Check sheet for the modelled part. Datum: model origin and axes. Units: mm. Face numbers are marked on the shaded views. A direction names the side the tool comes from. Round coordinates to 2 decimals unless told otherwise and drop trailing zeros. Order: outer loops, then holes, each group sorted by start corner. A loop starts at its lowest first (then second) coordinate and runs counter-clockwise, first axis right, second up.
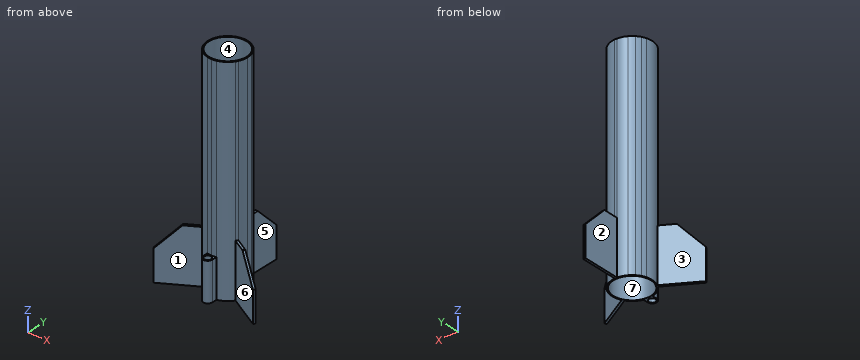
from build123d import *

# Parameters (mm, degrees)
F0_R     = 12.25
F1_DEPTH = 140
F2_DEPTH = 35
F3_SIZE  = 15
F4_COUNT = 3
F0_R_2   = 2.25
F5_DEPTH = 25
F6_START = 62
F0_R_3   = 11
F6_DEPTH = 2


with BuildPart() as f1:
    # F0 (on Top) → F1 (new body)
    with BuildSketch(Plane.XY):
        with BuildLine():
            ThreePointArc((3, -12.6491106407), (10.1980390272, -8.0622577483), (13, 0))
            ThreePointArc((13, 0), (9.4538352006, 8.9232841488), (0.75, 12.9783473524))
            ThreePointArc((0.75, 12.9783473524), (0, 13), (-0.75, 12.9783473524))
            ThreePointArc((-0.75, 12.9783473524), (-12.9501843924, 1.1369803002), (-3, -12.6491106407))
            ThreePointArc((-3, -12.6491106407), (-1.5102254126, -12.9119796779), (2.58e-08, -13))
            ThreePointArc((2.58e-08, -13), (1.5102254382, -12.9119796749), (3, -12.6491106407))
        make_face()
        Circle(F0_R, mode=Mode.SUBTRACT)
    extrude(amount=F1_DEPTH)

    # F0 (on Top) → F2 (join)
    with BuildSketch(Plane.XY):
        with BuildLine():
            ThreePointArc((-0.75, 12.9783473524), (0, 13), (0.75, 12.9783473524))
            Line((0.75, 12.9783473524), (0.75, 37.9783473524))
            Line((0.75, 37.9783473524), (-0.75, 37.9783473524))
            Line((-0.75, 37.9783473524), (-0.75, 12.9783473524))
        make_face()
    extrude(amount=F2_DEPTH)

    # F3
    f3_edges = [f1.edges().sort_by_distance(p)[0] for p in [
        (0, 37.978347, 35),
    ]]
    chamfer(f3_edges, length=F3_SIZE)


with BuildPart() as f4_1:
    # F4: instance of F1
    add(f1.part.rotate(Axis((0, 0, 140), (0, 0, 1)), 1 * 360 / F4_COUNT))


with BuildPart() as f4_2:
    # F4: instance of F1
    add(f1.part.rotate(Axis((0, 0, 140), (0, 0, 1)), 2 * 360 / F4_COUNT))


with BuildPart() as f1_1:
    add(f1.part)

    add(f4_1.part)  # F5 merges F4_1

    add(f4_2.part)  # F5 merges F4_2
    # F0 (on Top) → F5 (join)
    with BuildSketch(Plane.XY):
        with BuildLine():
            ThreePointArc((3, -16), (2.1213203527, -13.8786796655), (2.58e-08, -13))
            ThreePointArc((2.58e-08, -13), (-2.1213203345, -13.8786796473), (-3, -16))
            ThreePointArc((-3, -16), (0, -19), (3, -16))
        make_face()
        with Locations((0, -16)):
            Circle(F0_R_2, mode=Mode.SUBTRACT)
        with BuildLine():
            Line((3, -16), (3, -12.6491106407))
            ThreePointArc((3, -12.6491106407), (1.5102254382, -12.9119796749), (2.58e-08, -13))
            ThreePointArc((2.58e-08, -13), (2.1213203527, -13.8786796655), (3, -16))
        make_face()
        with BuildLine():
            ThreePointArc((-3, -16), (-2.1213203345, -13.8786796473), (2.58e-08, -13))
            ThreePointArc((2.58e-08, -13), (-1.5102254126, -12.9119796779), (-3, -12.6491106407))
            Line((-3, -12.6491106407), (-3, -16))
        make_face()
    extrude(amount=F5_DEPTH)

    # F0 (on Top) → F6 (join)
    with BuildSketch(Plane.XY.offset(F6_START)):
        Circle(F0_R)
        Circle(F0_R_3, mode=Mode.SUBTRACT)
    extrude(amount=F6_DEPTH)


solid = f1_1.part
1) Gauge pin test, flat ends, axial feed: pin 1 (20 mm diameter, centred on y = 26.5, z = 23.5, fed in from +X); pin 2 (5 mm diameter, centred on x = -14.5, y = -10, fed in from +Z); pin 3 (1.8 mm diameter, centred on x = -0.5, y = -16, fed in from +Z); pin 4 (1 mm diameter, centred on y = -14, z = 16.5, fed in from +X). Record the tip position at first contact, or that the pin passes through.
2) Scan lines: line 1 (Y direction, x = 1, z = 22.5); line 2 (X direction, y = 1, z = 9); line 3 (Y direction, x = -2, z = 11). Record each from-to range of solid material in increasing order.
3) Set-up check for the marked faces 1, 2, 3 and 4: record each of +Z, -Z, +X, -X, +Y, -Y from which the full face is reachable in a straight line by a thin tool's end or side.
4) Sectioned sample at D-D on y = 16.5. Record the cut outline in (x, z).
5) Sectioned sample at C-C on y = -3. Record the cut outline in (x, z).
6) Sectioned sample at B-B on x = 6. Record the cut outline in (y, z), and give its area (3 significant figures).
7) Sectioned sample at A-A on z = 52. Record the cut outline in (x, y).
8) Draft check along Y on the marked faces 5, 6 and 7. Enter one of: pulls with the +Y half, pulls with the -Y half, needs draft (parallel to the pull), parting line crosses it, or undercut.
Values found:
1. pin 1: stops at x = 0.75
1. pin 2: stops at z = 35
1. pin 3: passes through
1. pin 4: stops at x = 26.61
2. line 1: y = -18.83 to -18.02, -13.98 to -12.21, 12.21 to 12.96
2. line 2: x = -12.96 to -12.21, 12.21 to 12.96
2. line 3: y = -18.24 to -17.03, -14.97 to -12.09, 12.09 to 12.85
3. face 1: +Z, -Z, -Y
3. face 2: +Z, -Z, -X, +Y
3. face 3: +Z, -Z, -X
3. face 4: +Z
4. outline: (-0.75, 0) - (0.75, 0) - (0.75, 35) - (-0.75, 35) - close
5. outline: (-12.65, 0) - (-11.88, 0) - (-11.88, 62) - (-10.58, 62) - (-10.58, 64) - (-11.88, 64) - (-11.88, 140) - (-12.65, 140) - close; (10.58, 62) - (11.88, 62) - (11.88, 0) - (12.65, 0) - (12.65, 140) - (11.88, 140) - (11.88, 64) - (10.58, 64) - close
6. outline: (-11.53, 0) - (-10.68, 0) - (-10.68, 62) - (-9.22, 62) - (-9.22, 64) - (-10.68, 64) - (-10.68, 140) - (-11.53, 140) - close; (9.22, 62) - (10.68, 62) - (10.68, 0) - (11.53, 0) - (11.53, 140) - (10.68, 140) - (10.68, 64) - (9.22, 64) - close
6. area: 245 mm2
7. outline: circle Ø26 at (0, 0); hole circle Ø24.5 at (0, 0)
8. face 5: needs draft
8. face 6: pulls with the -Y half
8. face 7: undercut
